Source: CAD feature listing. Evaluate the final solid. Frame: model axes, mm. A direction names the side the tool comes from. Round coordinates to 2 decimals unless told otherwise and drop trailing zeros. Loops run counter-clockwise (first coordinate to the right, second up) from the corner with the lowest first, then second, coordinate; pieces in that order, holes last.
(1) First-contact query: pin 1 Ø4 at (x, y) = (616.5, -198) entering from +Z; pin 2 Ø4 at (y, z) = (-117.5, 21) entering from +X; pin 3 Ø5 at (y, z) = (-1421.5, 43) entering from -X. Flat tips, straight axial feed; report the tip coordinate or a pass-through.
(2) Mould query, pull axis Y, two halves, no side actions, for faces 1 (the flat face through (204, -1759, 89)), 2 (the cylindrical face through (-882.426, -1005.86, 43.877)), 3 (the cylindrical face through (375.35, 15.27, 2.28)). Classes: pulls with the +Y half, pulls with the -Y half, needs draft (parallel to the pull), parting line crosses it, or undercut.
(3) Section B-B, the plane x = 0. Return the cut outline in (y, z).
(4) Set-up query: faces 4 (the cylindrical face through (-270.34, -31.56, 53.19)), 5 (the flat face through (867, -1103, 0)). Return all of +Z, -Z, +X, -X, +Y, -Y with unobstructed straight access to the full face (end or side cutting, diameter ignored); none if empty.
(5) Material intervals for probe 1 along X at (y, z) = (-890, 60.5); probe 2 along Y at (x, z) = (0, 39); probe 3 along X at (y, z) = (-193, 28), sorted ascending.
(6) Section A-A, the plane y = -890. Return the cut outline in (x, z), plus the area to 3 significant figures.
(7) Section C-C, the plane z = 41.5. Return the cut outline in (x, y), plus the area to 3 significant figures.
```python
from build123d import *

# Parameters (mm, degrees)
F2_W     = 1953.7661696216
F2_H     = 27.2181874708
F3_DEPTH = 900


with BuildPart() as f1:
    # F0 (on Right) → F1 (revolve)
    with BuildSketch(Plane.YZ):
        with BuildLine():
            Line((4.5, 90), (0, 90))
            Line((0, 90), (0, 0))
            Line((0, 0), (90, 0))
            Line((90, 0), (90, 4.5))
            ThreePointArc((90, 4.5), (88.3890872965, 8.3890872965), (84.5, 10))
            Line((84.5, 10), (21, 10))
            ThreePointArc((21, 10), (13.2218254069, 13.2218254069), (10, 21))
            Line((10, 21), (10, 84.5))
            ThreePointArc((10, 84.5), (8.3890872965, 88.3890872965), (4.5, 90))
        make_face()
    revolve(axis=Axis((0, -890, 43.0200174451), (0, 0, 1)))

    # F2 (on Right) → F3 (cut, symmetric)
    with BuildSketch(Plane.YZ):
        with Locations((-897.6354291663, 102.6090937354)):
            Rectangle(F2_W, F2_H)
    extrude(amount=F3_DEPTH, both=True, mode=Mode.SUBTRACT)


solid = f1.part
```
Output values:
1. pin 1: stops at z = 10
1. pin 2: stops at x = 465.11
1. pin 3: stops at x = -728.12
2. face 1: needs draft
2. face 2: undercut
2. face 3: parting line crosses it
3. outline: (-1870, 0) - (-1780, 0) - (-1780, 89) - (-1787.66, 89) arc R5.5 ccw to (-1790, 84.5) - (-1790, 21) arc R11 cw to (-1801, 10) - (-1864.5, 10) arc R5.5 ccw to (-1870, 4.5) - close; (0, 0) - (90, 0) - (90, 4.5) arc R5.5 ccw to (84.5, 10) - (21, 10) arc R11 cw to (10, 21) - (10, 84.5) arc R5.5 ccw to (7.66, 89) - (0, 89) - close
4. face 4: +Z
4. face 5: -Z, +X, -X, +Y, -Y
5. probe 1: x = -900 to -890, 890 to 900
5. probe 2: y = -1790 to -1780, 0 to 10
5. probe 3: x = -569.38 to -553.44, 553.44 to 569.38
6. outline: (-980, 0) - (-890, 0) - (-890, 89) - (-897.66, 89) arc R5.5 ccw to (-900, 84.5) - (-900, 21) arc R11 cw to (-911, 10) - (-974.5, 10) arc R5.5 ccw to (-980, 4.5) - close; (890, 0) - (980, 0) - (980, 4.5) arc R5.5 ccw to (974.5, 10) - (911, 10) arc R11 cw to (900, 21) - (900, 84.5) arc R5.5 ccw to (897.66, 89) - (890, 89) - close
6. area: 3,410 mm2
7. outline: circle Ø1800 at (0, -890); hole circle Ø1780 at (0, -890)
7. area: 56,200 mm2
